from build123d import *

# Parameters (mm, degrees)
ESBO_O1_W                = 16.8
ESBO_O1_H                = 12.8
RESSALTO_EXTRUS_O1_DEPTH = 15
RESSALTO_EXTRUS_O2_DEPTH = 16.8
CASCA1_T                 = -1
ESBO_O5_R                = 24
CORTE_EXTRUS_O1_DEPTH    = 22.8000001
RESSALTO_EXTRUS_O3_DEPTH = 2
RESSALTO_EXTRUS_O4_DEPTH = 1


with BuildPart() as part:
    # Esboço1 → Ressalto-extrusão1 (new body)
    with BuildSketch(Plane.XY):
        Rectangle(ESBO_O1_W, ESBO_O1_H)
    extrude(amount=RESSALTO_EXTRUS_O1_DEPTH)

    # Esboço2 → Ressalto-extrusão2 (add, through all)
    with BuildSketch(Plane(origin=(8.4, 0, 0), x_dir=(0, 0, -1), z_dir=(1, 0, 0))):
        with BuildLine():
            Line((-25.102885683, -15.4), (-29, -13.15))
            add(Edge.make_bspline(
                [(-15, 6.4), (-24.5700068, 6.4), (-28.06930524, -8.749171672), (-29, -13.15)],
                knots=[0, 0, 0, 0, 1, 1, 1, 1], degree=3))
            Line((-15, 6.4), (-15, -6.4))
            add(Edge.make_bspline(
                [(-15, -6.4), (-18.032161103, -6.4), (-23.944769552, -12.297903221), (-25.102885683, -15.4)],
                knots=[0, 0, 0, 0, 1, 1, 1, 1], degree=3))
        make_face()
    extrude(amount=-RESSALTO_EXTRUS_O2_DEPTH)

    # Casca1
    casca1_openings = [part.faces().sort_by_distance(p)[0] for p in [
        (0, -14.275, 27.051442841),
        (0, 0, 0),
    ]]
    offset(amount=CASCA1_T, openings=casca1_openings)

    # Esboço5 → Corte-extrusão1 (cut, through all)
    with BuildSketch(Plane(origin=(0, 6.4, 0), x_dir=(1, 0, 0), z_dir=(0, 1, 0))):
        with Locations((16.15, 10.4)):
            Circle(ESBO_O5_R)
    extrude(amount=-CORTE_EXTRUS_O1_DEPTH, mode=Mode.SUBTRACT)

    # Esboço6 → Ressalto-extrusão3 (add)
    with BuildSketch(Plane.XZ.offset(6.4)):
        with BuildLine():
            Line((23, 25.6), (8.4, 25.6))
            Line((8.4, 25.6), (8.4, 15.6))
            Line((8.4, 15.6), (23, 15.6))
            ThreePointArc((23, 15.6), (28, 20.6), (23, 25.6))
        make_face()
        with BuildLine():
            Line((19, 22.25), (23, 22.25))
            ThreePointArc((23, 22.25), (24.65, 20.6), (23, 18.95))
            Line((23, 18.95), (19, 18.95))
            ThreePointArc((19, 18.95), (17.35, 20.6), (19, 22.25))
        make_face(mode=Mode.SUBTRACT)
    extrude(amount=-RESSALTO_EXTRUS_O3_DEPTH)

    # Esboço7 → Ressalto-extrusão4 (add)
    with BuildSketch(Plane.XZ.offset(6.4)):
        with BuildLine():
            Line((19, 25.6), (23, 25.6))
            ThreePointArc((23, 25.6), (28, 20.6), (23, 15.6))
            Line((23, 15.6), (19, 15.6))
            ThreePointArc((19, 15.6), (14, 20.6), (19, 25.6))
        make_face()
        with BuildLine():
            Line((19, 18.95), (23, 18.95))
            ThreePointArc((23, 18.95), (24.65, 20.6), (23, 22.25))
            Line((23, 22.25), (19, 22.25))
            ThreePointArc((19, 22.25), (17.35, 20.6), (19, 18.95))
        make_face(mode=Mode.SUBTRACT)
    extrude(amount=RESSALTO_EXTRUS_O4_DEPTH)


solid = part.part
Verification items for the finished model (mm, model axes). A direction names the side the tool comes from. Give positions to 0.01 mm unless a question says otherwise; leave off trailing zeros. Loops run counter-clockwise (first coordinate to the right, second up) from the corner with the lowest first, then second, coordinate; pieces in that order, holes last.
1) Sectioned sample at B-B, the plane x = 16. Enter the section's corners in (y, z).
2) Set-up check for faces 4 (the flat face through (16, -4.4, 21)), 5 (the flat face through (21, -6, 18.95)), 6 (the flat face through (-2, 5.4, 9)), 7 (the flat face through (16, -6, 15.6)): record each of +Z, -Z, +X, -X, +Y, -Y from which the full face is reachable in a straight line by a thin tool's end or side.
3) Depth check by flat-ended pin: pin 1 Ø5 at (x, y) = (2.5, -4) entering from +Z; pin 2 Ø16.5 at (x, z) = (-1.5, 5) entering from -Y; pin 3 Ø1.5 at (x, y) = (13.5, -5.5) entering from +Z; pin 4 Ø1 at (x, z) = (19, 21.5) entering from +Y. Enter the tip coordinate at first touch or a pass-through.
4) Thickness scan on line 1 along Y through (x, z) = (-2.5, 7.75); line 2 along X through (y, z) = (-3.5, 19.5); line 3 along X through (y, z) = (3, 2.25). Record the ranges inside material, lowest first.
5) Sectioned sample at D-D, the plane z = 9. Enter the section's corners in (x, y), then the cut area to 3 significant figures.
6) Sectioned sample at C-C, the plane z = 20.6. Count the separate pieces of the cut face and the enclosed holes in it, then the cut area to 3 significant figures.
7) Draft check along X on faces 1 (the cylindrical face through (1.27, -5.66, 8.43)), 2 (the flat face through (-8, 0, 0)), 3 (the cylindrical face through (14, -6.9, 20.5)). Enter one of: pulls with the +X half, pulls with the -X half, needs draft (parallel to the pull), parting line crosses it, or undercut.
8) Sectioned sample at A-A, the plane z = 14. Enter the section's corners in (x, y), then the cut area to 3 significant figures.
Answers:
1. outline: (-7.4, 16.6) - (-6.4, 16.6) - (-6.4, 15.6) - (-4.4, 15.6) - (-4.4, 25.6) - (-6.4, 25.6) - (-6.4, 24.6) - (-7.4, 24.6) - close
2. face 4: +Z, -Z, +X, +Y
2. face 5: +Y, -Y
2. face 6: -Z
2. face 7: -Z, +X, +Y, -Y
3. pin 1: stops at z = 27.21
3. pin 2: stops at y = -6.4
3. pin 3: stops at z = 25.6
3. pin 4: passes through
4. line 1: y = -6.4 to -5.4, 5.4 to 6.4
4. line 2: x = -8.4 to -7.4, 7.4 to 8.4
4. line 3: x = -8.4 to -7.4
5. outline: (-8.4, -6.4) - (2.02, -6.4) - (2.02, -5.4) - (-7.4, -5.4) - (-7.4, 5.4) - (2.02, 5.4) - (2.02, 6.4) - (-8.4, 6.4) - close
5. area: 31.6 mm2
6. separate pieces: 2
6. enclosed holes: 1
6. area: 98.4 mm2
7. face 1: pulls with the +X half
7. face 2: needs draft
7. face 3: undercut
8. outline: (-8.4, -6.4) - (8.4, -6.4) - (8.4, 6.4) - (-8.4, 6.4) - close; hole (-7.4, -5.4) - (7.4, -5.4) - (7.4, 5.4) - (-7.4, 5.4) - close
8. area: 55.2 mm2
